Input: part model. Units: mm. Frame: model coordinates. A direction names the side the tool comes from. Round coordinates to 2 decimals unless told otherwise and drop trailing zeros. Loops run counter-clockwise (first coordinate to the right, second up) from the corner with the lowest first, then second, coordinate; pieces in that order, holes last. Notation, with made-up numbers: (-8.5, 59.25) -> (50.5, 59.25) arc R16 ccw to (50.5, 74.25) -> close; hole circle Ø3 at (-24, 60). An arc over 180 degrees is marked (long way). Answer as a JSON object with one key per item and string values.
```python
from build123d import *

# Parameters (mm, degrees)
SKETCH1_R           = 1.5
BOSS_EXTRUDE1_DEPTH = 21


with BuildPart() as part:
    # Sketch1 → Boss-Extrude1 (new body)
    with BuildSketch(Plane(origin=(0, 0, 0), x_dir=(1, 0, 0), z_dir=(0, 1, 0))):
        with BuildLine():
            Line((0, 20), (-30, 20))
            Line((-30, 20), (-30, 30))
            Line((-30, 30), (30, 30))
            Line((30, 30), (30, -30))
            Line((30, -30), (-30, -30))
            Line((-30, -30), (-30, -20))
            Line((-30, -20), (0, -20))
            ThreePointArc((0, -20), (20, 0), (0, 20))
        make_face()
        with Locations(Location((-23.5, 23.5, 0), (0, 0, 90))):
            Circle(SKETCH1_R, mode=Mode.SUBTRACT)
        with Locations(Location((23.5, 23.5, 0), (0, 0, 90))):
            Circle(SKETCH1_R, mode=Mode.SUBTRACT)
        with Locations(Location((-23.5, -23.5, 0), (0, 0, 90))):
            Circle(SKETCH1_R, mode=Mode.SUBTRACT)
        with Locations(Location((23.5, -23.5, 0), (0, 0, 90))):
            Circle(SKETCH1_R, mode=Mode.SUBTRACT)
    extrude(amount=BOSS_EXTRUDE1_DEPTH)


solid = part.part
```
1) Ray query, probe 1 along Z at (x, y) = (23.5, 16.75); probe 2 along Z at (x, y) = (-6.5, 5). Return the intervals inside material, ascending.
Output:
{"probe 1": "z = -30 to -25, -22 to 22, 25 to 30", "probe 2": "z = -30 to -20, 20 to 30"}
2) Section C-C, the plane x = -23.5. Output: boundary loops of the cut face in (y, z), plus the area to 3 significant figures.
Output:
{"outline": "(0, -30) -> (21, -30) -> (21, -25) -> (0, -25) -> close; (0, -22) -> (21, -22) -> (21, -20) -> (0, -20) -> close; (0, 20) -> (21, 20) -> (21, 22) -> (0, 22) -> close; (0, 25) -> (21, 25) -> (21, 30) -> (0, 30) -> close", "area": "294 mm^2"}
3) Reachability of faces 1 (the face through (-15, 10, 20)), 2 (the face through (-24.987, 10.353, -23.305)) from +Z, -Z, +X, -X, +Y, -Y: full face, straight path, thin tool, end or side. Return the list, or none.
Output:
{"face 1": "-X, +Y, -Y", "face 2": "+Y, -Y"}
4) Section B-B, the plane x = 23.5. Output: boundary loops of the cut face in (y, z), plus the area to 3 significant figures.
Output:
{"outline": "(0, -30) -> (21, -30) -> (21, -25) -> (0, -25) -> close; (0, -22) -> (21, -22) -> (21, 22) -> (0, 22) -> close; (0, 25) -> (21, 25) -> (21, 30) -> (0, 30) -> close", "area": "1,130 mm^2"}
5) Contact query for flat-ended pins moving along their axis: P1, Ø4, axis at y = 17, z = -5, coming from the -X side (3 decimals); P2, Ø2, axis at y = 11.5, z = 13, coming from the -X side. Output: stop coordinate, or through.
Output:
{"P1": "stops at x = 18.735", "P2": "stops at x = 14.28"}
6) Draft query along Z for faces 3 (the face through (-30, 10, 25)), 4 (the face through (0, 10, -30)), 5 (the face through (22.49, 10.35, 24.61)). Return one class per face: +Z half, -Z half, draft (parallel to the pull), parting line (faces both ways), or undercut.
Output:
{"face 3": "draft", "face 4": "-Z half", "face 5": "undercut"}
7) Section D-D, the plane y = 17.25. Output: boundary loops of the cut face in (x, z), plus the area to 3 significant figures.
Output:
{"outline": "(-30, -30) -> (30, -30) -> (30, 30) -> (-30, 30) -> (-30, 20) -> (0, 20) arc R20 cw to (0, -20) -> (-30, -20) -> close; hole circle Ø3 at (-23.5, -23.5); hole circle Ø3 at (-23.5, 23.5); hole circle Ø3 at (23.5, -23.5); hole circle Ø3 at (23.5, 23.5)", "area": "1,740 mm^2"}
8) Section A-A, the plane z = 23.5. Output: boundary loops of the cut face in (x, y).
Output:
{"outline": "(-30, 0) -> (-25, 0) -> (-25, 21) -> (-30, 21) -> close; (-22, 0) -> (22, 0) -> (22, 21) -> (-22, 21) -> close; (25, 0) -> (30, 0) -> (30, 21) -> (25, 21) -> close"}
